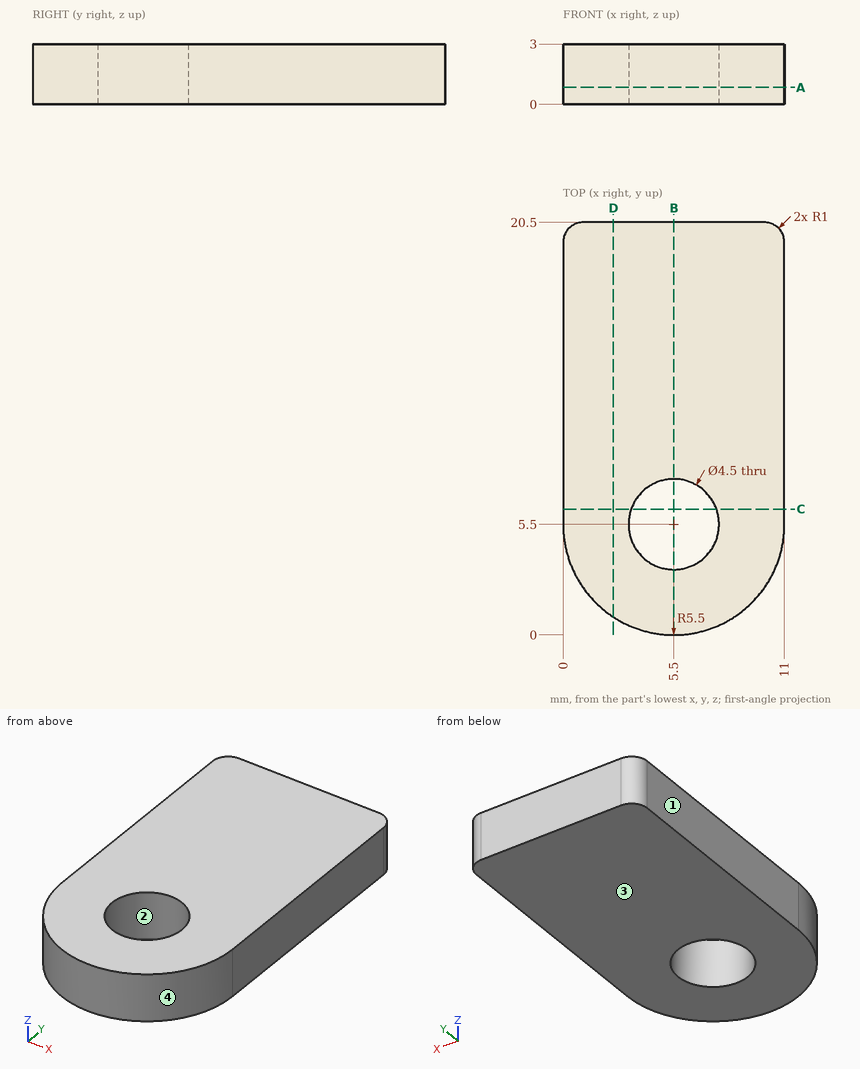
Input: dimensioned drawing with shaded views. Units: mm. Origin: part minimum x, y, z. Give positions to 0.01 mm unless a question says otherwise; leave off trailing zeros. Loops run counter-clockwise (first coordinate to the right, second up) from the corner with the lowest first, then second, coordinate; pieces in that order, holes last. Notation, with made-up numbers: M -1,58 L 35,58 A25 cw 35,74 Z; hole C 30,81 d11. An arc over 180 degrees is marked long. Put each result on its own line as item: value. Start each with the question number.
1) Pull-direction query (X, two-part tool) for the marked faces 1, 2, 3 and 4; classes: pulls with the +X half, pulls with the -X half, needs draft (parallel to the pull), parting line crosses it, or undercut.
2) Cut plane B-B (x = 5.5). Output: boundary loops of the cut face in (y, z), then the cut area to 3 significant figures.
3) Cut plane C-C (y = 6.25). Output: boundary loops of the cut face in (x, z), then the cut area to 3 significant figures.
4) Contact query for flat-ended pins moving along their axis: pin 1 (5 mm diameter, centred on x = 3, y = 3.5, fed in from -Z); pin 2 (1.5 mm diameter, centred on x = 8, z = 2, fed in from -Y). Output: stop coordinate, or through.
5) Ray query, line 1 along Y through (x, z) = (5.5, 1.9); line 2 along X through (y, z) = (6.25, 1.9); line 3 along X through (y, z) = (7.5, 1.05). Return the intervals inside material, ascending.
6) Cut plane D-D (x = 2.5). Output: boundary loops of the cut face in (y, z), then the cut area to 3 significant figures.
7) Cut plane A-A (z = 0.85). Output: boundary loops of the cut face in (x, y).
Verdict:
1. face 1: pulls with the -X half
1. face 2: undercut
1. face 3: needs draft
1. face 4: parting line crosses it
2. outline: M 0,0 L 3.25,0 L 3.25,3 L 0,3 Z; M 7.75,0 L 20.5,0 L 20.5,3 L 7.75,3 Z
2. area: 48.0 mm2
3. outline: M 0,0 L 3.38,0 L 3.38,3 L 0,3 Z; M 7.62,0 L 11,0 L 11,3 L 7.62,3 Z
3. area: 20.3 mm2
4. pin 1: z = 0
4. pin 2: y = 0.29
5. line 1: 0 to 3.25, 7.75 to 20.5
5. line 2: 0 to 3.38, 7.62 to 11
5. line 3: 0 to 4.47, 6.53 to 11
6. outline: M 0.89,0 L 20.5,0 L 20.5,3 L 0.89,3 Z
6. area: 58.8 mm2
7. outline: M 0,5.5 A5.5 ccw 11,5.5 L 11,19.5 A1 ccw 10,20.5 L 1,20.5 A1 ccw 0,19.5 Z; hole C 5.5,5.5 d4.5
